Geometry: final body of the model. Coordinates: model frame, mm. Coordinates: 2 decimals unless noted, no trailing zeros. Write each loop counter-clockwise with the first axis right and the second up, starting at its lowest first coordinate (ties: lowest second). Pieces come first, ordered by that corner, then holes. Notation, with made-up numbers: (35, -19.75) - (88, -19.75) arc R30 ccw to (88, 4.25) - close; hole circle Ø5 at (-25.75, 81). An arc over 180 degrees is marked (long way). Answer as a JSON object with one key per item and string values. Group by question number.
Item 1: Line query: line 1 along Y through (x, z) = (8.71, 0.8) (3 decimals); line 2 along X through (y, z) = (7, 0.2); line 3 along X through (y, z) = (6.5, 1.45). Output: solid intervals per line, ascending. Write a range as from..to.
Item 2: Mould query, pull axis Y, two halves, no side actions, for faces 1 (the cylindrical face through (10.096, -7.75, 0.74)), 2 (the flat face through (0, 0, 1.5)). Classes: pulls with the +Y half, pulls with the -Y half, needs draft (parallel to the pull), parting line crosses it, or undercut.
Item 3: Section A-A on y = -7.75. Return loops of the section in (x, z), and give its area (3 significant figures).
Item 4: Section C-C on z = 0.9. State how many separate pieces and enclosed holes the cut face has, and give its area (3 significant figures).
Item 5: Section B-B on x = 8.71. Return loops of the section in (y, z) (3 decimals).
Item 6: First-contact query: pin 1 Ø2.5 at (x, y) = (-8.71, -7.175) entering from -Z. Flat tip, straight axial feed; report the tip coordinate or a pass-through.
```python
from build123d import *

# Parameters (mm, degrees)
F0_R     = 1.5
F1_DEPTH = 1.5


with BuildPart() as f1:
    # F0 (on Top) → F1 (new body)
    with BuildSketch(Plane.XY):
        with BuildLine():
            add(Edge.make_bspline(
                [(-5.5561550838, 5.6573497621), (-4.0955413133, 3.5522743128), (-3.2797986642, 3.3143495675), (0, 3.173440462)],
                knots=[0, 0, 0, 0, 6.0861042323, 6.0861042323, 6.0861042323, 6.0861042323], degree=3))
            ThreePointArc((-5.5561550838, 5.6573497621), (-11.1647533144, 9.6698318912), (-7.2436210565, 3.9969923231))
            add(Edge.make_bspline(
                [(-7.2436210565, 3.9969923231), (-6.2028751709, 2.9064782429), (-5.828993395, 2.9744568747), (-5.7950043119, 0)],
                knots=[0, 0, 0, 0, 4.2514042508, 4.2514042508, 4.2514042508, 4.2514042508], degree=3))
            add(Edge.make_bspline(
                [(-7.2436210565, -3.9969923231), (-6.2028751709, -2.9064782429), (-5.828993395, -2.9744568747), (-5.7950043119, 0)],
                knots=[0, 0, 0, 0, 4.2514042508, 4.2514042508, 4.2514042508, 4.2514042508], degree=3))
            ThreePointArc((-7.2436210565, -3.9969923231), (-11.1647533144, -9.6698318912), (-5.5561550838, -5.6573497621))
            add(Edge.make_bspline(
                [(-5.5561550838, -5.6573497621), (-4.0955413133, -3.5522743128), (-3.2797986642, -3.3143495675), (0, -3.173440462)],
                knots=[0, 0, 0, 0, 6.0861042323, 6.0861042323, 6.0861042323, 6.0861042323], degree=3))
            add(Edge.make_bspline(
                [(5.5561550838, -5.6573497621), (4.0955413133, -3.5522743128), (3.2797986642, -3.3143495675), (0, -3.173440462)],
                knots=[0, 0, 0, 0, 6.0861042323, 6.0861042323, 6.0861042323, 6.0861042323], degree=3))
            ThreePointArc((5.5561550838, -5.6573497621), (11.1647533144, -9.6698318912), (7.2436210565, -3.9969923231))
            add(Edge.make_bspline(
                [(7.2436210565, -3.9969923231), (6.2028751709, -2.9064782429), (5.828993395, -2.9744568747), (5.7950043119, 0)],
                knots=[0, 0, 0, 0, 4.2514042508, 4.2514042508, 4.2514042508, 4.2514042508], degree=3))
            add(Edge.make_bspline(
                [(7.2436210565, 3.9969923231), (6.2028751709, 2.9064782429), (5.828993395, 2.9744568747), (5.7950043119, 0)],
                knots=[0, 0, 0, 0, 4.2514042508, 4.2514042508, 4.2514042508, 4.2514042508], degree=3))
            ThreePointArc((7.2436210565, 3.9969923231), (11.1647533144, 9.6698318912), (5.5561550838, 5.6573497621))
            add(Edge.make_bspline(
                [(5.5561550838, 5.6573497621), (4.0955413133, 3.5522743128), (3.2797986642, 3.3143495675), (0, 3.173440462)],
                knots=[0, 0, 0, 0, 6.0861042323, 6.0861042323, 6.0861042323, 6.0861042323], degree=3))
        make_face()
        with Locations((-8.71, -7.175)):
            Circle(F0_R, mode=Mode.SUBTRACT)
        with Locations((8.71, -7.175)):
            Circle(F0_R, mode=Mode.SUBTRACT)
        with Locations((-8.71, 7.175)):
            Circle(F0_R, mode=Mode.SUBTRACT)
        with Locations((8.71, 7.175)):
            Circle(F0_R, mode=Mode.SUBTRACT)
    extrude(amount=F1_DEPTH)


solid = f1.part
```
Checks:
{
 "1": {"line 1": "-10.675..-8.675, -5.675..-3.675, 3.675..5.675, 8.675..10.675", "line 2": "-12.21..-10.2, -7.22..-5.21, 5.21..7.22, 10.2..12.21", "line 3": "-12.14..-10.05, -7.37..-5.28, 5.28..7.37, 10.05..12.14"},
 "2": {"face 1": "undercut", "face 2": "needs draft"},
 "3": {"outline": "(-12.16, 0) - (-10.1, 0) - (-10.1, 1.5) - (-12.16, 1.5) - close; (-7.32, 0) - (-5.26, 0) - (-5.26, 1.5) - (-7.32, 1.5) - close; (5.26, 0) - (7.32, 0) - (7.32, 1.5) - (5.26, 1.5) - close; (10.1, 0) - (12.16, 0) - (12.16, 1.5) - (10.1, 1.5) - close", "area": "12.4 mm^2"},
 "4": {"separate pieces": "1", "enclosed holes": "4", "area": "223 mm^2"},
 "5": {"outline": "(-10.675, 0) - (-8.675, 0) - (-8.675, 1.5) - (-10.675, 1.5) - close; (-5.675, 0) - (-3.675, 0) - (-3.675, 1.5) - (-5.675, 1.5) - close; (3.675, 0) - (5.675, 0) - (5.675, 1.5) - (3.675, 1.5) - close; (8.675, 0) - (10.675, 0) - (10.675, 1.5) - (8.675, 1.5) - close"},
 "6": {"pin 1": "through"}
}
